from build123d import *

# Parameters (mm, degrees)
BOSS_EXTRUDE1_DEPTH = 584.2
FILLET1_R           = 1.5875


with BuildPart() as part:
    # Sketch1 → Boss-Extrude1 (new body, symmetric)
    with BuildSketch(Plane(origin=(0, 0, 0), x_dir=(0, 0, -1), z_dir=(1, 0, 0))):
        with BuildLine():
            Line((-1.5875, 28.575), (-7.9375, 28.575))
            Line((-7.9375, 28.575), (-7.9375, -1.5875))
            ThreePointArc((-7.9375, -1.5875), (0, -9.525), (7.9375, -1.5875))
            Line((7.9375, -1.5875), (7.9375, 28.575))
            Line((7.9375, 28.575), (1.5875, 28.575))
            Line((1.5875, 28.575), (1.5875, 0))
            Line((1.5875, 0), (-1.5875, 0))
            Line((-1.5875, 0), (-1.5875, 28.575))
        make_face()
    extrude(amount=BOSS_EXTRUDE1_DEPTH, both=True)

    # Fillet1
    fillet1_edges = [part.edges().sort_by_distance(p)[0] for p in [
        (0, 28.575, -7.9375),
        (0, 28.575, 7.9375),
    ]]
    fillet(fillet1_edges, radius=FILLET1_R)


solid = part.part
Could you check a few things on this model? Use its own coordinates, in mm. A direction names the side the tool comes from. Round coordinates to 2 decimals unless told otherwise and drop trailing zeros. Write each loop counter-clockwise with the first axis right and the second up, starting at its lowest first coordinate (ties: lowest second). Pieces come first, ordered by that corner, then holes. Notation, with made-up numbers: (43, -26.75) - (74, -26.75) arc R12 ccw to (74, -6.75) - close; hole circle Ø4 at (-25.75, 13.5). An arc over 180 degrees is marked (long way). Put each result on its own line as item: value. Start each with the question number.
(1) I need wall thicknesses on probe 1 along Z at (x, y) = (-136, 1.5); probe 2 along Y at (x, z) = (388.5, 5) (3 decimals); probe 3 along Y at (x, z) = (197, 0.5). Which ranges of each line are inside material? Lowest first, please.
(2) Will this pin go through, and if not, where does the flat tip stop? pin 1 (2.5 mm diameter, centred on x = -282, z = 0, fed in from +Y).
(3) I want a section at A-A, the plane y = 19. Please give me the cut outline in (x, z), plus the area to 3 significant figures.
(4) For faces 1 (the flat face through (8, 14, -1.588)), 2 (the flat face through (8, 13, 7.938)), which set-ups out of +Z, -Z, +X, -X, +Y, -Y let a thin tool reach every point of the face, with its end or its side?
Here are the results:
1. probe 1: z = -7.94 to -1.59, 1.59 to 7.94
1. probe 2: y = -7.752 to 28.575
1. probe 3: y = -9.51 to 0
2. pin 1: stops at y = 0
3. outline: (-584.2, -7.94) - (584.2, -7.94) - (584.2, -1.59) - (-584.2, -1.59) - close; (-584.2, 1.59) - (584.2, 1.59) - (584.2, 7.94) - (-584.2, 7.94) - close
3. area: 14,800 mm^2
4. face 1: +X, -X, +Y
4. face 2: +Z, +X, -X, +Y, -Y
